Build history of the part. All positions in model axes, mm. Round coordinates to 2 decimals unless told otherwise and drop trailing zeros. Write each loop counter-clockwise with the first axis right and the second up, starting at its lowest first coordinate (ties: lowest second). Pieces come first, ordered by that corner, then holes.
1) Saw through at B-B (z = -135). Write the cut outline in (x, y), plus the area to 3 significant figures.
2) Pull direction Z, two halves, no side cores. Call faces 1 (the flat face through (-2, 5, 150)), 2 (the flat face through (-2, 0, -2)), 3 (the cylindrical face through (-66.354, 4.93, 116.318)): +Z half, -Z half, draft (parallel to the pull), parting line (faces both ways), or undercut.
3) Wall check: probe 1 along X at (y, z) = (6.5, 116.5); probe 2 along Z at (x, y) = (-70, 7); probe 3 along Z at (x, y) = (70.5, 2.5). Give the ranges that are in metal, low to high.
4) Flat gauge pin, fed straight in: pin 1 (7.5 mm diameter, centred on x = 65.5, z = 96.5, fed in from -Y). Where does the tip first touch, or does it go through?
5) Saw through at A-A (x = 135). Write the cut outline in (y, z).
from build123d import *

# Parameters (mm, degrees)
SKETCH1_W                           = 300
SKETCH1_H                           = 300
BOSS_EXTRUDE1_DEPTH                 = 10
TAPPED_HOLE_FOR_M8X1_25_HELICOIL1_D = 8.3
M8_CLEARANCE_HOLE2_D                = 9


with BuildPart() as part:
    # Sketch1 → Boss-Extrude1 (new body)
    with BuildSketch(Plane(origin=(0, 0, 0), x_dir=(1, 0, 0), z_dir=(0, 1, 0))):
        Rectangle(SKETCH1_W, SKETCH1_H)
    extrude(amount=BOSS_EXTRUDE1_DEPTH)

    # Tapped Hole for M8x1.25 Helicoil1 (through all)
    with Locations(Plane(origin=(0, 10, 0), x_dir=(1, 0, 0), z_dir=(0, 1, 0))):
        with Locations((70.5, 116.5), (70.5, 96.5), (65.5, -96.5), (65.5, -116.5), (-65.5, 116.5), (-65.5, 96.5), (-70.5, -96.5), (-70.5, -116.5)):
            Hole(TAPPED_HOLE_FOR_M8X1_25_HELICOIL1_D / 2)

    # M8 Clearance Hole2 (through all)
    with Locations(Plane(origin=(0, 10, 0), x_dir=(1, 0, 0), z_dir=(0, 1, 0))):
        with Locations((-135, -135), (-135, 135), (135, 135), (135, -135)):
            Hole(M8_CLEARANCE_HOLE2_D / 2)


solid = part.part
Evaluation:
1. outline: (-150, 0) - (-139.5, 0) - (-139.5, 10) - (-150, 10) - close; (-130.5, 0) - (130.5, 0) - (130.5, 10) - (-130.5, 10) - close; (139.5, 0) - (150, 0) - (150, 10) - (139.5, 10) - close
1. area: 2,820 mm2
2. face 1: +Z half
2. face 2: draft
2. face 3: undercut
3. probe 1: x = -150 to -74.65, -66.35 to 61.35, 69.65 to 150
3. probe 2: z = -150 to 92.38, 100.62 to 112.38, 120.62 to 150
3. probe 3: z = -150 to -120.65, -112.35 to -100.65, -92.35 to 150
4. pin 1: passes through
5. outline: (0, -150) - (10, -150) - (10, -139.5) - (0, -139.5) - close; (0, -130.5) - (10, -130.5) - (10, 130.5) - (0, 130.5) - close; (0, 139.5) - (10, 139.5) - (10, 150) - (0, 150) - close
